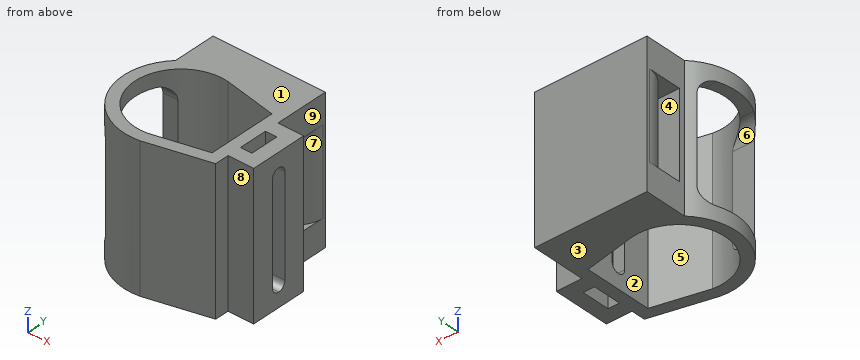
from build123d import *

# Parameters (mm, degrees)
SALIENTE_EXTRUIR1_DEPTH = 50
SALIENTE_EXTRUIR2_DEPTH = 50
CORTAR_EXTRUIR12_REACH  = 81.477
CROQUIS12_W             = 40
CROQUIS12_H             = 5
REDONDEO1_R             = 2.5
CROQUIS16_W             = 40
CROQUIS16_H             = 26.726230184
CORTAR_EXTRUIR17_DEPTH  = 20
REDONDEO2_R             = 5
CORTAR_EXTRUIR18_REACH  = 77.626
CROQUIS21_W             = 30
CROQUIS21_H             = 3
REDONDEO3_R             = 9


with BuildPart() as part:
    # Croquis3 → Saliente-Extruir1 (new body)
    with BuildSketch(Plane.XY):
        with BuildLine():
            Line((-4.157247249, -24.2640649), (-26.215773458, -29.447511872))
            ThreePointArc((-26.215773458, -29.447511872), (-47.164183017, -18.638090647), (-43.521067646, 4.65154569))
            Line((-43.521067646, 4.65154569), (-43.521067646, 19.65154569))
            Line((-43.521067646, 19.65154569), (-4.157247249, 19.65154569))
            Line((-4.157247249, 19.65154569), (-4.157247249, -24.2640649))
        make_face()
        with BuildLine():
            Line((-8.157247249, 2.82108494), (-26.731262437, 6.441781026))
            ThreePointArc((-26.731262437, 6.441781026), (-45.345288804, -9.402744466), (-26.961453667, -25.513783269))
            Line((-26.961453667, -25.513783269), (-8.157247249, -21.095056202))
            Line((-8.157247249, -21.095056202), (-8.157247249, 2.82108494))
        make_face(mode=Mode.SUBTRACT)
    extrude(amount=SALIENTE_EXTRUIR1_DEPTH)

    # Croquis11 → Saliente-Extruir2 (add)
    with BuildSketch(Plane(origin=(0, 0, 0), x_dir=(-1, 0, 0), z_dir=(0, 0, -1))):
        Polygon((-4.842752751, -19.306259605), (-4.842752751, 0.693740395), (4.157247249, 0.693740395), (4.157247249, -4.306259605), (0.157247249, -4.306259605), (0.157247249, -14.306259605), (4.157247249, -14.306259605), (4.157247249, -19.306259605), align=None)
    extrude(amount=-SALIENTE_EXTRUIR2_DEPTH)

    # Cortar-Extruir12: up to this face of the body (flat: up to its plane)
    cortar_extruir12_end = Plane(part.part.faces().sort_by_distance((-8.157247249, -9.136985631, 25))[0])
    # Croquis12 → Cortar-Extruir12 (cut, up to the picked face)
    with BuildSketch(Plane(origin=(4.842752751, 0, 0), x_dir=(0, 0, -1), z_dir=(1, 0, 0)), mode=Mode.PRIVATE) as cortar_extruir12_sk1:
        with Locations((-25, -9.306259605)):
            Rectangle(CROQUIS12_W, CROQUIS12_H)
    cortar_extruir12_tool1 = split(extrude(cortar_extruir12_sk1.sketch, amount=-CORTAR_EXTRUIR12_REACH, mode=Mode.PRIVATE), bisect_by=cortar_extruir12_end, keep=Keep.BOTH, mode=Mode.PRIVATE)
    add(cortar_extruir12_tool1.solids().sort_by(Axis((4.842753, -9.30626, 25), (-1, 0, 0)))[0], mode=Mode.SUBTRACT)

    # Redondeo1
    redondeo1_edges = [part.edges().sort_by_distance(p)[0] for p in [
        (2.342752751, -6.806259605, 5),
        (2.342752751, -6.806259605, 45),
        (-6.157247249, -11.806259605, 5),
        (-6.157247249, -6.806259605, 5),
        (-6.157247249, -11.806259605, 45),
        (-6.157247249, -6.806259605, 45),
        (2.342752751, -11.806259605, 5),
        (2.342752751, -11.806259605, 45),
    ]]
    fillet(redondeo1_edges, radius=REDONDEO1_R - 0.0001)  # a hair under: the kernel refuses the full size

    # Croquis16 → Cortar-Extruir17 (cut, symmetric)
    with BuildSketch(Plane.ZY.offset(48.157247249)):
        with Locations((25, -11.305962539)):
            Rectangle(CROQUIS16_W, CROQUIS16_H)
    extrude(amount=CORTAR_EXTRUIR17_DEPTH, both=True, mode=Mode.SUBTRACT)

    # Redondeo2
    redondeo2_edges = [part.edges().sort_by_distance(p)[0] for p in [
        (-43.072694771, 2.057152553, 45),
        (-38.635693074, -24.669077631, 45),
        (-38.635693074, -24.669077631, 5),
        (-43.072694771, 2.057152553, 5),
    ]]
    fillet(redondeo2_edges, radius=REDONDEO2_R)

    # Croquis21 → Cortar-Extruir18 (cut, up to next)
    with BuildSketch(Plane.ZY.offset(43.521067646), mode=Mode.PRIVATE) as cortar_extruir18_sk1:
        with Locations((25, 8.15154569)):
            Rectangle(CROQUIS21_W, CROQUIS21_H)
    cortar_extruir18_tool1 = extrude(cortar_extruir18_sk1.sketch, amount=-CORTAR_EXTRUIR18_REACH, mode=Mode.PRIVATE) & part.part
    add(cortar_extruir18_tool1.solids().sort_by_distance((-43.521068, 8.151546, 25))[0], mode=Mode.SUBTRACT)

    # Redondeo3
    redondeo3_edges = [part.edges().sort_by_distance(p)[0] for p in [
        (-43.521067646, 9.65154569, 25),
        (-4.157247249, 9.65154569, 25),
    ]]
    fillet(redondeo3_edges, radius=REDONDEO3_R)


solid = part.part
The listing builds one solid part. Answer for the finished solid, in the listing's coordinates (mm). Face numbers are marked on the shaded views. A direction names the side the tool comes from. Round coordinates to 2 decimals unless told otherwise and drop trailing zeros. Write each loop counter-clockwise with the first axis right and the second up, starting at its lowest first coordinate (ties: lowest second). Pieces come first, ordered by that corner, then holes. Notation, with made-up numbers: (25, 35.25) - (80, 35.25) arc R19 ccw to (80, 53.25) - close; hole circle Ø9 at (74, 58.5). An arc over 180 degrees is marked (long way). Use one line per item in the form item = value. Start each with the question number.
Item 1: A cutting plane is placed at A-A (x = -3). Write down the section's boundary in (y, z).
Item 2: Determine the mould class of the marked faces 1, 2, 3 and 4 for opening direction Z: +Z half, -Z half, draft (parallel to the pull), parting line (faces both ways), or undercut.
Item 3: A cutting plane is placed at C-C (y = -8). Write down the section's boundary in (x, z).
Item 4: Find the intervals of material crossed by line 1 (X direction, y = -6.5, z = 32); line 2 (Y direction, x = 0.5, z = 23.5); line 3 (Y direction, x = -1, z = 14.5), in increasing order. Write a range as [from, to].
Item 5: A tool of negligible diameter and unlimited length cuts with its end or side. For the marked faces 5, 6, 7, 8 and 9, from which of +Z, -Z, +X, -X, +Y, -Y can it reach the whole face along a straight path? Write none if from no direction.
Item 6: A cutting plane is placed at D-D (y = -2). Write down the section's boundary in (x, z), plus the area to 3 significant figures.
Item 7: Flat-ended cylindrical pins translate along their axes: pin 1 Ø1.5 at (x, z) = (-22, 9.5) entering from -Y; pin 2 Ø12 at (y, z) = (-13, 20.5) entering from -X; pin 3 Ø3 at (x, z) = (-2.5, 33.5) entering from +Y. Find the tip coordinate at first contact, or state that the pin passes through.
Item 8: A cutting plane is placed at B-B (z = 47.5). Write down the section's boundary in (x, y), plus the area to 3 significant figures.
The answers:
q1.outline = (-19.31, 0) - (-14.31, 0) - (-14.31, 50) - (-19.31, 50) - close; (-4.31, 0) - (0.69, 0) - (0.69, 50) - (-4.31, 50) - close
q2.face_1 = +Z half
q2.face_2 = draft
q2.face_3 = -Z half
q2.face_4 = undercut
q3.outline = (-49.29, 0) - (-45.27, 0) - (-45.27, 5) - (-49.29, 5) - close; (-49.29, 45) - (-45.27, 45) - (-45.27, 50) - (-49.29, 50) - close; (-8.16, 0) - (-4.16, 0) - (-4.16, 5.37) - (-8.16, 5.37) - close; (-8.16, 44.63) - (-4.16, 44.63) - (-4.16, 50) - (-8.16, 50) - close; (-0.16, 0) - (4.84, 0) - (4.84, 5.37) - (-0.16, 5.37) - close; (-0.16, 44.63) - (4.84, 44.63) - (4.84, 50) - (-0.16, 50) - close
q4.line_1 = [-8.16, -4.16], [-0.16, 4.84]
q4.line_2 = [-19.31, -11.81], [-6.81, 0.69]
q4.line_3 = [-19.31, -14.31], [-4.31, 0.69]
q5.face_5 = +Z, -Z
q5.face_6 = -X
q5.face_7 = +X
q5.face_8 = +Z, -Z, +X, -Y
q5.face_9 = +Z, -Z, +X, +Y
q6.outline = (-47.89, 0) - (-43.49, 0) - (-43.49, 5.09) - (-47.89, 5.09) - close; (-47.89, 44.91) - (-43.49, 44.91) - (-43.49, 50) - (-47.89, 50) - close; (-8.16, 0) - (4.84, 0) - (4.84, 50) - (-8.16, 50) - close
q6.area = 695 mm^2
q7.pin_1 = -28.63
q7.pin_2 = -8.16
q7.pin_3 = 0.69
q8.outline = (-43.52, 4.65) arc R20.15 ccw to (-26.22, -29.45) - (-4.16, -24.26) - (-4.16, -19.31) - (4.84, -19.31) - (4.84, 0.69) - (-4.16, 0.69) - (-4.16, 19.65) - (-43.52, 19.65) - close; hole (-26.96, -25.51) - (-8.16, -21.1) - (-8.16, 2.82) - (-26.73, 6.44) arc R16.15 ccw (long way) to start; hole (-4.16, -14.31) - (-0.16, -14.31) - (-0.16, -4.31) - (-4.16, -4.31) - close
q8.area = 1,100 mm^2
